Part print with two shaded views. Sizes in mm from the minimum x, y, z corner. A direction names the side the tool comes from. Coordinates: 2 decimals unless noted, no trailing zeros. Write each loop counter-clockwise with the first axis right and the second up, starting at its lowest first coordinate (ties: lowest second). Pieces come first, ordered by that corner, then holes. Notation, with made-up numbers: (-20.75, 40) - (35.25, 40) arc R23 ccw to (35.25, 77) - close; hole circle Ø4 at (-33.75, -25). An arc over 180 degrees is marked (long way). Answer in a Markdown table with one row per item. Add a question column.
Q1. Band-saw the part on B-B (x = 82). List the corners of the cut face in (y, z), and give its area (3 significant figures).
Q2. Band-saw the part on C-C (y = 60.5). List the corners of the cut face in (x, z), and give its area (3 significant figures).
Q3. Band-saw the part on A-A (y = 29). List the corners of the cut face in (x, z).
Q4. 3-axis set-ups, long thin cutter, end or side, ignore diameter. For the marked faces 1 and 2: which of +Z, -Z, +X, -X, +Y, -Y reach the whole face in a straight line?
Q5. Band-saw the part on D-D (z = 39). List the corners of the cut face in (x, y).
Q6. Drill centre lines: line 1 along Z through (x, y) = (65.5, 91.5); line 2 along X through (y, z) = (32.5, 30.5). Where is each one in solid material? Low to high. Write a range as from..to.
Q7. Pin check, flat tips, straight feed: pin 1 (1.5 mm diameter, centred on x = 95, z = 23.5, fed in from -Y); pin 2 (0.9 mm diameter, centred on x = 95, z = 46, fed in from +Y); pin 3 (8 mm diameter, centred on y = 10.5, z = 12, fed in from -X); pin 4 (8 mm diameter, centred on y = 13, z = 23.5, fed in from -X). Stop position of each tip, or through.
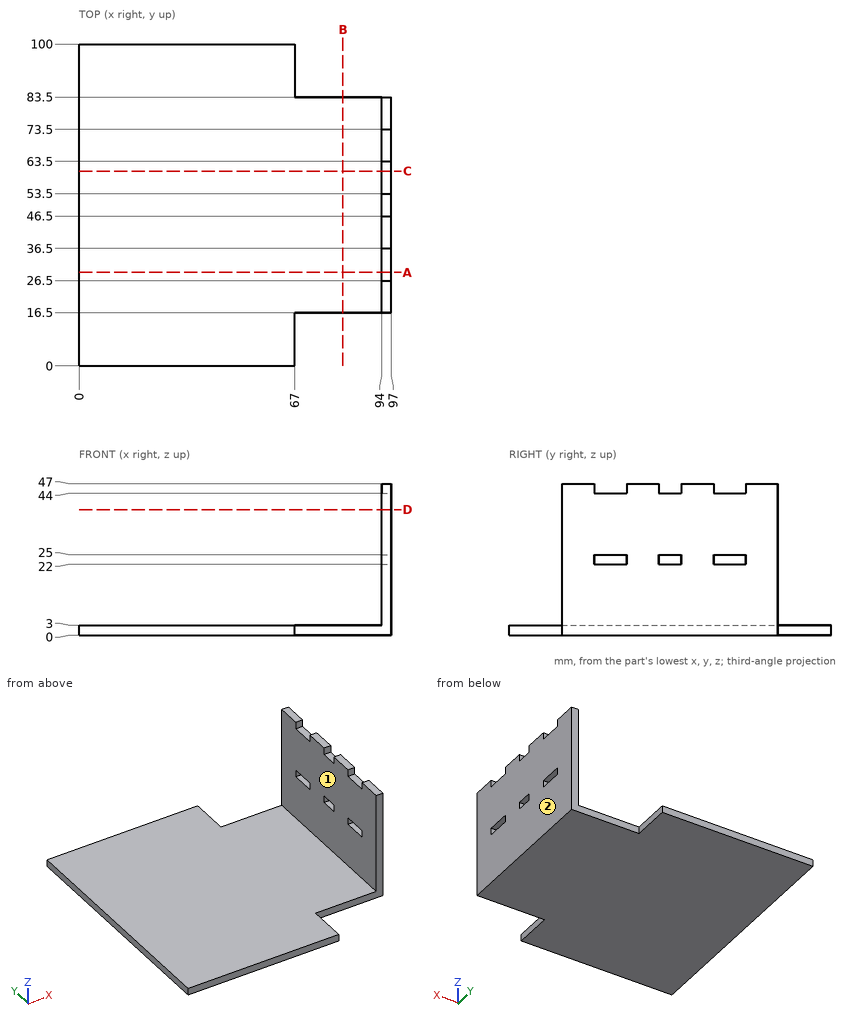
Checked values:
| question | item | result |
|---|---|---|
| 1 | outline | (16.5, 0) - (83.5, 0) - (83.5, 3) - (16.5, 3) - close |
| 1 | area | 201 mm² |
| 2 | outline | (0, 0) - (97, 0) - (97, 47) - (94, 47) - (94, 3) - (0, 3) - close |
| 2 | area | 423 mm² |
| 3 | outline | (0, 0) - (97, 0) - (97, 22) - (94, 22) - (94, 3) - (0, 3) - close; (94, 25) - (97, 25) - (97, 44) - (94, 44) - close |
| 4 | face 1 | +Z, -X, +Y, -Y |
| 4 | face 2 | +Z, -Z, +X, +Y, -Y |
| 5 | outline | (94, 16.5) - (97, 16.5) - (97, 83.5) - (94, 83.5) - close |
| 6 | line 1 | z = 0..3 |
| 6 | line 2 | x = 94..97 |
| 7 | pin 1 | stops at y = 16.5 |
| 7 | pin 2 | stops at y = 83.5 |
| 7 | pin 3 | passes through |
| 7 | pin 4 | stops at x = 94 |
